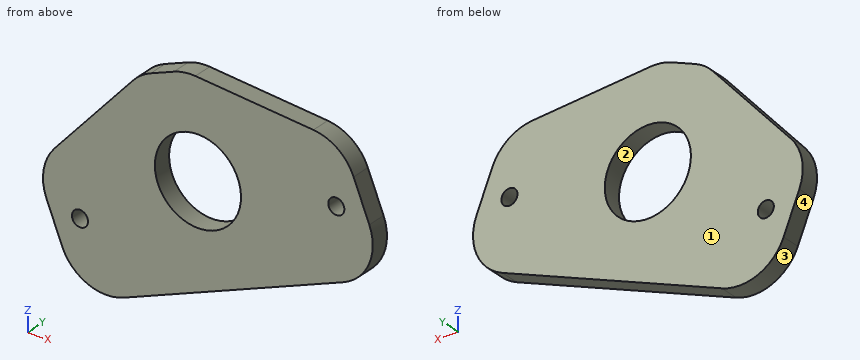
```python
from build123d import *

# Parameters (mm, degrees)
SKETCH_1_R          = 1.7
SKETCH_1_R_2        = 9.1
EXTRUDE_1_DEPTH     = 4
CUT_EXTRUDE_1_DEPTH = 4
FILLET_1_R          = 10


with BuildPart() as part:
    # 草图1 → 凸台-拉伸1 (new body)
    with BuildSketch(Plane(origin=(0, 0, 0), x_dir=(1, 0, 0), z_dir=(0, 1, 0))):
        Polygon((-126.240398859, 38.128502465), (-191.110616974, 64.43163539), (-206.140978645, 27.362939325), (-141.27076053, 1.059806399), align=None)
        with Locations(Location((-136.961696425, 27.654734478, 0), (0, 0, 270))):
            Circle(SKETCH_1_R, mode=Mode.SUBTRACT)
        with Locations(Location((-191.102800779, 48.48323248, 0), (0, 0, 270))):
            Circle(SKETCH_1_R, mode=Mode.SUBTRACT)
        with Locations(Location((-166.190688752, 32.745720895, 0), (0, 0, 270))):
            Circle(SKETCH_1_R_2, mode=Mode.SUBTRACT)
    extrude(amount=EXTRUDE_1_DEPTH)

    # 草图2 → 切除-拉伸1 (cut)
    with BuildSketch(Plane(origin=(0, 4, 0), x_dir=(1, 0, 0), z_dir=(0, 1, 0))):
        Polygon((-135.634374903, 14.960567424), (-169.07228258, 12.332577653), (-141.27076053, 1.059806399), align=None)
        Polygon((-200.504593019, 41.263700349), (-178.339456596, 16.090168071), (-206.140978645, 27.362939325), align=None)
    extrude(amount=-CUT_EXTRUDE_1_DEPTH, mode=Mode.SUBTRACT)

    # 圆角1
    fillet_1_edges = [part.edges().sort_by_distance(p)[0] for p in [
        (-135.634374903, 2, -14.960567424),
        (-169.07228258, 2, -12.332577653),
        (-200.504593019, 2, -41.263700349),
        (-178.339456596, 2, -16.090168071),
        (-191.110616974, 2, -64.43163539),
        (-126.240398859, 2, -38.128502465),
    ]]
    fillet(fillet_1_edges, radius=FILLET_1_R)


solid = part.part
```
Can you work these out from the model? Positions are in its coordinate system, mm. Face numbers are marked on the shaded views. Coordinates: 2 decimals unless noted, no trailing zeros. Loops run counter-clockwise (first coordinate to the right, second up) from the corner with the lowest first, then second, coordinate; pieces in that order, holes last.
Item 1: I'm going to push flat-ended pins straight in: pin 1 (1.5 mm diameter, centred on y = 1.5, z = -41.5, fed in from +X); pin 2 (1 mm diameter, centred on x = -138.5, y = 0.5, fed in from -Z). Where does each tip first touch, or does it pass through?
Answers below:
pin 1: stops at x = -133.44
pin 2: stops at z = -43.3
Item 2: Suppose I cut it at D-D (y = 1.3). Please give me the cut outline in (x, z), then the cut area to 3 significant figures.
Answers below:
outline: (-198.18, -46.99) - (-194.87, -55.16) arc R10 ccw to (-181.84, -60.67) - (-135.51, -41.89) arc R10 ccw to (-130, -28.86) - (-133.31, -20.69) arc R10 ccw to (-141.8, -14.48) - (-166.72, -12.52) arc R10 ccw to (-171.26, -13.22) - (-176.15, -15.2) arc R10 ccw to (-179.9, -17.86) - (-196.42, -36.63) arc R10 ccw to start; hole circle Ø3.4 at (-191.1, -48.48); hole circle Ø18.2 at (-166.19, -32.75); hole circle Ø3.4 at (-136.96, -27.65)
area: 2,020 mm2
Item 3: Suppose I cut it at A-A (z = -40). Please give me the cut outline in (x, y), then the cut area to 3 significant figures.
Answers below:
outline: (-198.38, 0) - (-171.68, 0) - (-171.68, 4) - (-198.38, 4) - close; (-160.7, 0) - (-132.52, 0) - (-132.52, 4) - (-160.7, 4) - close
area: 219 mm2
Item 4: If we mould it in two halves opening along X, with no side actions, what happens to the marked faces 1, 2, 3 and 4? For each: released by +X, released by -X, zero draft, split by the parting line, or undercut.
Answers below:
face 1: zero draft
face 2: undercut
face 3: split by the parting line
face 4: released by -X
Item 5: Suppose I cut it at C-C (z = -27.5). Please give me the cut outline in (x, y).
Answers below:
outline: (-188.39, 0) - (-173.63, 0) - (-173.63, 4) - (-188.39, 4) - close; (-158.75, 0) - (-138.65, 0) - (-138.65, 4) - (-158.75, 4) - close; (-135.27, 0) - (-130.55, 0) - (-130.55, 4) - (-135.27, 4) - close
Item 6: Suppose I cut it at B-B (x = -160). Please give me the cut outline in (y, z).
Answers below:
outline: (0, -51.82) - (4, -51.82) - (4, -39.42) - (0, -39.42) - close; (0, -26.08) - (4, -26.08) - (4, -13.05) - (0, -13.05) - close
Item 7: Please list where these lines run through material, in increasing order: L1, parallel to Z at x = -169, y = 2.3; L2, parallel to Z at x = -136.5, y = 2.8; L3, parallel to X at y = 3.3, z = -49.5 (3 decimals).
Answers below:
L1: z = -55.47 to -41.4, -24.09 to -12.6
L2: z = -42.29 to -29.29, -26.02 to -16.51
L3: x = -197.165 to -192.465, -189.74 to -154.285
